For this review, take the finished solid that the model builds, in its own axes (mm). Coordinates: 2 decimals unless noted, no trailing zeros.
Autodesk Inventor part; units mm, degrees
ref_plane "YZ Plane" through (0, 0, 0) normal (1, 0, 0) x (0, 1, 0)
ref_plane "XZ Plane" through (0, 0, 0) normal (0, 1, 0) x (-1, 0, 0)
ref_plane "XY Plane" through (0, 0, 0) normal (0, 0, 1) x (1, 0, 0)
ref_plane "Work Plane1" through (45.1427, 7.5316, -333.0131) normal (-0.0001, 0, -1) x (0, -1, 0)
sketch "Sketch1" plane through (45.1427, 7.5316, -333.0131) normal (-0.0001, 0, -1) x (0, -1, 0)
  line L0 (333.4019, -100.965) -> (333.4019, -89.027)
  line L1 (117.2921, 3.175) -> (326.375, 3.175)
  line L2 (326.375, 3.175) -> (326.375, -108.4168)
  line L3 (326.375, -108.4168) -> (117.2921, -108.4168)
  line L4 (117.2921, -108.4168) -> (117.2921, 3.175)
  circle A0 centre (673.1, -9.525) radius 2.667
  circle A1 centre (647.7, -9.525) radius 2.667
  circle A2 centre (622.3, -9.525) radius 2.667
  circle A3 centre (596.9, -9.525) radius 2.667
  circle A4 centre (571.5, -9.525) radius 2.667
  circle A5 centre (546.1, -9.525) radius 2.667
  circle A6 centre (520.7, -9.525) radius 2.667
  circle A7 centre (495.3, -9.525) radius 2.667
  circle A8 centre (469.9, -9.525) radius 2.667
  circle A9 centre (444.5, -9.525) radius 2.667
  circle A10 centre (419.1, -9.525) radius 2.667
  circle A11 centre (393.7, -9.525) radius 2.667
  circle A12 centre (368.3, -9.525) radius 2.667
  circle A13 centre (342.9, -9.525) radius 2.667
  circle A14 centre (317.5, -9.525) radius 2.667
  circle A15 centre (292.1, -9.525) radius 2.667
  circle A16 centre (266.7, -9.525) radius 2.667
  circle A17 centre (241.3, -9.525) radius 2.667
  circle A18 centre (215.9, -9.525) radius 2.667
  circle A19 centre (190.5, -9.525) radius 2.667
  circle A20 centre (165.1, -9.525) radius 2.667
  circle A21 centre (139.7, -9.525) radius 2.667
  line L5 (692.3329, -15.875) -> (692.3329, -0.762)
  line L6 (120.4671, -0.762) -> (692.3329, -0.762)
  line L7 (120.4671, -0.762) -> (120.4671, -15.875)
  line L8 (120.4671, -15.875) -> (692.3329, -15.875)
  line L9 (121.2291, -672.465) -> (136.3421, -672.465)
  line L10 (136.3421, -672.465) -> (136.3421, -19.685)
  line L11 (136.3421, -19.685) -> (121.2291, -19.685)
  line L12 (121.2291, -672.465) -> (121.2291, -19.685)
  circle A22 centre (129.9921, -663.575) radius 2.667
  circle A23 centre (129.9921, -638.175) radius 2.667
  circle A24 centre (129.9921, -612.775) radius 2.667
  circle A25 centre (129.9921, -587.375) radius 2.667
  circle A26 centre (129.9921, -561.975) radius 2.667
  circle A27 centre (129.9921, -536.575) radius 2.667
  circle A28 centre (129.9921, -511.175) radius 2.667
  circle A29 centre (129.9921, -485.775) radius 2.667
  circle A30 centre (129.9921, -460.375) radius 2.667
  circle A31 centre (129.9921, -434.975) radius 2.667
  circle A32 centre (129.9921, -409.575) radius 2.667
  circle A33 centre (129.9921, -384.175) radius 2.667
  circle A34 centre (129.9921, -358.775) radius 2.667
  circle A35 centre (129.9921, -333.375) radius 2.667
  circle A36 centre (129.9921, -307.975) radius 2.667
  circle A37 centre (129.9921, -282.575) radius 2.667
  circle A38 centre (129.9921, -257.175) radius 2.667
  circle A39 centre (129.9921, -231.775) radius 2.667
  circle A40 centre (129.9921, -206.375) radius 2.667
  circle A41 centre (129.9921, -180.975) radius 2.667
  circle A42 centre (129.9921, -155.575) radius 2.667
  circle A43 centre (129.9921, -130.175) radius 2.667
  circle A44 centre (129.9921, -104.775) radius 2.667
  circle A45 centre (129.9921, -79.375) radius 2.667
  circle A46 centre (129.9921, -53.975) radius 2.667
  circle A47 centre (129.9921, -28.575) radius 2.667
  circle A48 centre (180.3669, -28.575) radius 2.667
  circle A49 centre (180.3669, -53.975) radius 2.667
  circle A50 centre (180.3669, -79.375) radius 2.667
  circle A51 centre (180.3669, -104.775) radius 2.667
  circle A52 centre (180.3669, -130.175) radius 2.667
  circle A53 centre (180.3669, -155.575) radius 2.667
  circle A54 centre (180.3669, -180.975) radius 2.667
  circle A55 centre (180.3669, -206.375) radius 2.667
  circle A56 centre (180.3669, -231.775) radius 2.667
  circle A57 centre (180.3669, -257.175) radius 2.667
  circle A58 centre (180.3669, -282.575) radius 2.667
  line L13 (192.3049, -15.875) -> (174.0169, -15.875)
  line L14 (174.0169, -15.875) -> (174.0169, -292.1)
  line L15 (174.0169, -292.1) -> (177.1919, -295.275)
  line L16 (192.3049, -295.275) -> (177.1919, -295.275)
  line L17 (192.3049, -15.875) -> (192.3049, -295.275)
  circle A59 centre (219.1019, -72.39) radius 2.667
  circle A60 centre (244.5019, -72.39) radius 2.667
  circle A61 centre (269.9019, -72.39) radius 2.667
  circle A62 centre (295.3019, -72.39) radius 2.667
  circle A63 centre (320.7019, -72.39) radius 2.667
  circle A64 centre (346.1019, -72.39) radius 2.667
  line L18 (212.1169, -66.04) -> (212.1169, -84.328)
  line L19 (358.8019, -84.328) -> (212.1169, -84.328)
  line L20 (358.8019, -84.328) -> (358.8019, -69.215)
  line L21 (358.8019, -69.215) -> (355.6269, -66.04)
  line L22 (355.6269, -66.04) -> (212.1169, -66.04)
  point P0 (7.5323, 45.1616)
extrude "Extrusion1" add sketch "Sketch1" along normal blind 6.35 contours L1 L2 L6 L7 L8 L14 L3 L10 L11 L12 L4 | L2 L8 L7 L6 | L12 L11 L10 L3 | L2 L22 L18 L19 L3 L17 L8 | L2 L19 L18 L22 | L17 L3 L14 L8 | A14 | A15 | A16 | A17 | A18 | A19 | A20 | A21 | A44 | A45 | A46 | A47 | A48 | A49 | A50 | A51 | A59 | A60 | A61 | A62 | A63
sketch "Sketch2" plane through (45.1423, 7.5316, -339.3631) normal (-0.0001, 0, -1) x (-1, 0, 0.0001)
  circle A0 centre (-9.525, -673.1) radius 2.667
  circle A1 centre (-9.525, -647.7) radius 2.667
  circle A2 centre (-9.525, -622.3) radius 2.667
  circle A3 centre (-9.525, -596.9) radius 2.667
  circle A4 centre (-9.525, -571.5) radius 2.667
  circle A5 centre (-9.525, -546.1) radius 2.667
  circle A6 centre (-9.525, -520.7) radius 2.667
  circle A7 centre (-9.525, -495.3) radius 2.667
  circle A8 centre (-9.525, -469.9) radius 2.667
  circle A9 centre (-9.525, -444.5) radius 2.667
  circle A10 centre (-9.525, -419.1) radius 2.667
  circle A11 centre (-9.525, -393.7) radius 2.667
  circle A12 centre (-9.525, -368.3) radius 2.667
  circle A13 centre (-9.525, -342.9) radius 2.667
  circle A14 centre (-9.525, -317.5) radius 2.667
  circle A15 centre (-9.525, -292.1) radius 2.667
  circle A16 centre (-9.525, -266.7) radius 2.667
  circle A17 centre (-9.525, -241.3) radius 2.667
  circle A18 centre (-9.525, -215.9) radius 2.667
  circle A19 centre (-9.525, -190.5) radius 2.667
  circle A20 centre (-9.525, -165.1) radius 2.667
  circle A21 centre (-9.525, -139.7) radius 2.667
  line L0 (-15.875, -692.3329) -> (-0.762, -692.3329)
  line L1 (-0.762, -120.4671) -> (-0.762, -692.3329)
  line L2 (-0.762, -120.4671) -> (-15.875, -120.4671)
  line L3 (-15.875, -120.4671) -> (-15.875, -692.3329)
  circle A22 centre (-72.39, -219.1019) radius 2.667
  circle A23 centre (-72.39, -244.5019) radius 2.667
  circle A24 centre (-72.39, -269.9019) radius 2.667
  circle A25 centre (-72.39, -295.3019) radius 2.667
  circle A26 centre (-72.39, -320.7019) radius 2.667
  circle A27 centre (-72.39, -346.1019) radius 2.667
  line L4 (-66.04, -212.1169) -> (-84.328, -212.1169)
  line L5 (-84.328, -358.8019) -> (-84.328, -212.1169)
  line L6 (-84.328, -358.8019) -> (-69.215, -358.8019)
  line L7 (-69.215, -358.8019) -> (-66.04, -355.6269)
  line L8 (-66.04, -355.6269) -> (-66.04, -212.1169)
  circle A28 centre (-28.575, -180.3669) radius 2.667
  circle A29 centre (-53.975, -180.3669) radius 2.667
  circle A30 centre (-79.375, -180.3669) radius 2.667
  circle A31 centre (-104.775, -180.3669) radius 2.667
  circle A32 centre (-130.175, -180.3669) radius 2.667
  circle A33 centre (-155.575, -180.3669) radius 2.667
  circle A34 centre (-180.975, -180.3669) radius 2.667
  circle A35 centre (-206.375, -180.3669) radius 2.667
  circle A36 centre (-231.775, -180.3669) radius 2.667
  circle A37 centre (-257.175, -180.3669) radius 2.667
  circle A38 centre (-282.575, -180.3669) radius 2.667
  line L9 (-15.875, -192.3049) -> (-15.875, -174.0169)
  line L10 (-15.875, -174.0169) -> (-292.1, -174.0169)
  line L11 (-292.1, -174.0169) -> (-295.275, -177.1919)
  line L12 (-295.275, -192.3049) -> (-295.275, -177.1919)
  line L13 (-15.875, -192.3049) -> (-295.275, -192.3049)
  line L14 (-672.465, -121.2291) -> (-672.465, -136.3421)
  line L15 (-672.465, -136.3421) -> (-19.685, -136.3421)
  line L16 (-19.685, -136.3421) -> (-19.685, -121.2291)
  line L17 (-672.465, -121.2291) -> (-19.685, -121.2291)
  circle A39 centre (-663.575, -129.9921) radius 2.667
  circle A40 centre (-638.175, -129.9921) radius 2.667
  circle A41 centre (-612.775, -129.9921) radius 2.667
  circle A42 centre (-587.375, -129.9921) radius 2.667
  circle A43 centre (-561.975, -129.9921) radius 2.667
  circle A44 centre (-536.575, -129.9921) radius 2.667
  circle A45 centre (-511.175, -129.9921) radius 2.667
  circle A46 centre (-485.775, -129.9921) radius 2.667
  circle A47 centre (-460.375, -129.9921) radius 2.667
  circle A48 centre (-434.975, -129.9921) radius 2.667
  circle A49 centre (-409.575, -129.9921) radius 2.667
  circle A50 centre (-384.175, -129.9921) radius 2.667
  circle A51 centre (-358.775, -129.9921) radius 2.667
  circle A52 centre (-333.375, -129.9921) radius 2.667
  circle A53 centre (-307.975, -129.9921) radius 2.667
  circle A54 centre (-282.575, -129.9921) radius 2.667
  circle A55 centre (-257.175, -129.9921) radius 2.667
  circle A56 centre (-231.775, -129.9921) radius 2.667
  circle A57 centre (-206.375, -129.9921) radius 2.667
  circle A58 centre (-180.975, -129.9921) radius 2.667
  circle A59 centre (-155.575, -129.9921) radius 2.667
  circle A60 centre (-130.175, -129.9921) radius 2.667
  circle A61 centre (-104.775, -129.9921) radius 2.667
  circle A62 centre (-79.375, -129.9921) radius 2.667
  circle A63 centre (-53.975, -129.9921) radius 2.667
  circle A64 centre (-28.575, -129.9921) radius 2.667
  point P0 (45.1616, -7.5323)
extrude "Extrusion2" cut sketch "Sketch2" along normal mid plane 6.35 contours A14 | A15 | A16 | A17 | A18 | A19 | A20 | A21 | A22 | A23 | A24 | A25 | A26 | A28 | A29 | A30 | A31 | A61 | A62 | A63 | A64
properties part number "Aluminum Final Mounting Plate"
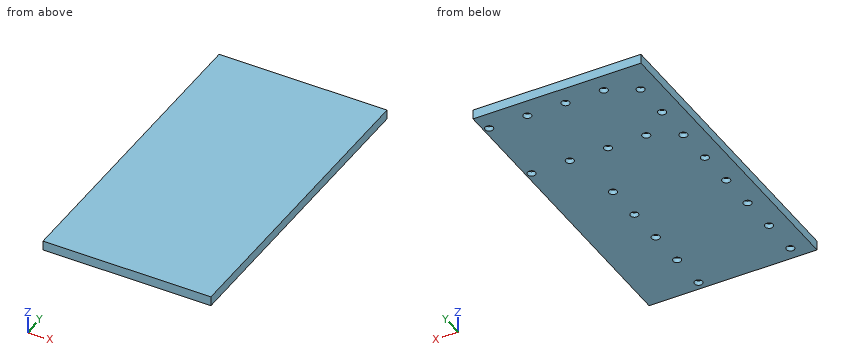
Q1. Clearance check with a flat-ended pin moving along its axis: pin 1 Ø2.5 at (x, y) = (55.5, -183) entering from -Z. State where the tip first meets the part, or that it passes through.
Ans:
pin 1: stops at z = -336.19
Q2. For probe 1 along Y at (x, z) = (117, -336.5); probe 2 along X at (y, z) = (-234, -336.5); probe 3 along Y at (x, z) = (119, -337), list the stretches that pass through material, from the lowest coordinate up.
Ans:
probe 1: y = -318.84 to -315.78, -310.56 to -290.38, -285.16 to -264.98, -259.76 to -239.58, -234.36 to -214.18, -208.96 to -109.76
probe 2: x = 41.97 to 52.01, 57.32 to 153.56
probe 3: y = -318.84 to -315.4, -310.94 to -290, -285.54 to -264.6, -260.14 to -239.2, -234.74 to -213.8, -209.34 to -109.76
Q3. Add section A-A (z = -337.5). Give the number of separate pieces and of enclosed holes in the cut face, then the cut area to 3 significant figures.
Ans:
separate pieces: 1
enclosed holes: 21
area: 22,900 mm2
